from build123d import *

# Parameters (mm, degrees)
SKETCH_1_R      = 4
SKETCH_1_R_2    = 1.5
EXTRUDE_1_DEPTH = 4


with BuildPart() as part:
    # 草图1 → 凸台-拉伸1 (new body)
    with BuildSketch(Plane.XY):
        with BuildLine():
            ThreePointArc((3.948047826, 9.187650318), (-5.50088728, 8.351062156), (-10, 0))
            add(Edge.make_bspline(
                [(-10, 0), (-10.890214237, -19.135341361), (75, -21.401956932)],
                knots=[0, 0, 0, 1, 1, 1], degree=2))
            add(Edge.make_bspline(
                [(160, 0), (160.890214237, -19.135341361), (75, -21.401956932)],
                knots=[0, 0, 0, 1, 1, 1], degree=2))
            ThreePointArc((160, 0), (155.415713455, 8.40654791), (145.865990446, 9.105490926))
            add(Edge.make_bspline(
                [(3.948047826, 9.187650318), (46.906488456, -20.373746255), (110.551742639, -16.70704022), (145.865990446, 9.105490926)],
                knots=[0.022448948, 0.022448948, 0.022448948, 0.022448948, 0.850781246, 0.850781246, 0.850781246, 0.850781246], degree=3))
        make_face()
        Circle(SKETCH_1_R, mode=Mode.SUBTRACT)
        with Locations((150, 0)):
            Circle(SKETCH_1_R_2, mode=Mode.SUBTRACT)
    extrude(amount=EXTRUDE_1_DEPTH)


solid = part.part
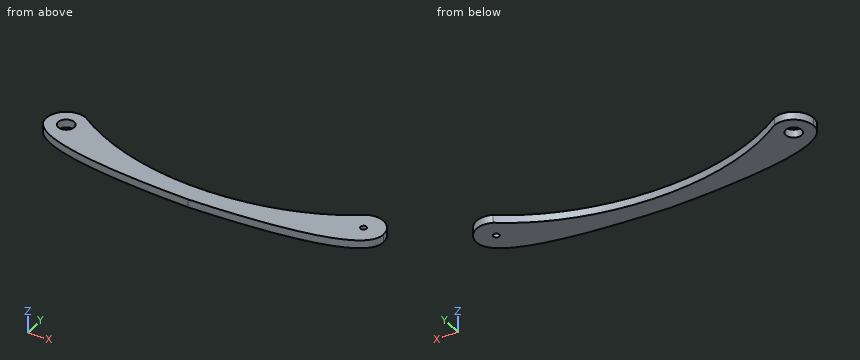
The model under review builds one solid part; all positions refer to its coordinate system, in mm. Coordinates: 2 decimals unless noted, no trailing zeros. Use a Markdown table: item, result. Add a question column.
1. Clearance check with flat-ended pins moving along their axes: pin 1 Ø2 at (y, z) = (-8, 2.5) entering from +X; pin 2 Ø1 at (y, z) = (-3, 3) entering from +X. State where each tip first meets the part, or that it passes through.
2. Add section A-A on z = 2.95. Give the number of separate pieces and of enclosed holes in the cut face, plus the area to 3 significant figures.
3. To check wall thickness, follow line 1 (X direction, y = 0.5, z = 1.85); line 2 (Y direction, x = 1, z = 1.1); line 3 (Y direction, x = 150, z = 2.4). State the ranges of each line that lie inside material, in increasing order.
Returned:
| question | item | result |
|---|---|---|
| 1 | pin 1 | stops at x = 156.86 |
| 1 | pin 2 | stops at x = 159.73 |
| 2 | separate pieces | 1 |
| 2 | enclosed holes | 2 |
| 2 | area | 2,360 mm² |
| 3 | line 1 | x = -9.99 to -3.97, 3.97 to 19.07, 131.42 to 148.59, 151.41 to 159.99 |
| 3 | line 2 | y = -11.76 to -3.87, 3.87 to 9.95 |
| 3 | line 3 | y = -11.32 to -1.5, 1.5 to 10 |
